Could you check a few things on this model? Use its own coordinates, in mm. A direction names the side the tool comes from. Give positions to 0.01 mm unless a question says otherwise; leave off trailing zeros. Loops run counter-clockwise (first coordinate to the right, second up) from the corner with the lowest first, then second, coordinate; pieces in that order, holes last. Notation, with made-up numbers: M -31,85 L 28,85 A34 ccw 28,118 Z; hole C -1,11 d6. An arc over 180 degrees is marked long. Write each question's results on one line, items separated by ' | '. Start each with the question number.
from build123d import *

# Parameters (mm, degrees)
SKETCH_1_W      = 23
SKETCH_1_H      = 20
SKETCH_1_H_2    = 12
SKETCH_1_R      = 1.5
SKETCH_1_W_2    = 19
SKETCH_1_R_2    = 1
EXTRUDE_1_DEPTH = 4
FILLET_1_R      = 3
CHAMFER_1_SIZE  = 15
FILLET_2_R      = 5


with BuildPart() as part:
    # 草图1 → 凸台-拉伸1 (new body)
    # profile 1 of 3: a face of its own
    with BuildSketch(Plane(origin=(0, 0, 0), x_dir=(1, 0, 0), z_dir=(0, 1, 0))):
        with Locations((51.5, 0)):
            Rectangle(SKETCH_1_W, SKETCH_1_H)
    # profile 2 of 3: a face of its own
    with BuildSketch(Plane(origin=(0, 0, 0), x_dir=(1, 0, 0), z_dir=(0, 1, 0))):
        with Locations((51.5, 16)):
            Rectangle(SKETCH_1_W, SKETCH_1_H_2)
        with Locations(Location((56, 18, 0), (0, 0, 270))):
            Circle(SKETCH_1_R, mode=Mode.SUBTRACT)
        with Locations(Location((48, 18, 0), (0, 0, 270))):
            Circle(SKETCH_1_R, mode=Mode.SUBTRACT)
    # profile 3 of 3: a face of its own
    with BuildSketch(Plane(origin=(0, 0, 0), x_dir=(1, 0, 0), z_dir=(0, 1, 0))):
        with Locations((30.5, 0)):
            Rectangle(SKETCH_1_W_2, SKETCH_1_H)
        with Locations(Location((24, -4, 0), (0, 0, 270))):
            Circle(SKETCH_1_R_2, mode=Mode.SUBTRACT)
        with Locations(Location((36, -4, 0), (0, 0, 270))):
            Circle(SKETCH_1_R_2, mode=Mode.SUBTRACT)
        with Locations(Location((24, 4, 0), (0, 0, 270))):
            Circle(SKETCH_1_R_2, mode=Mode.SUBTRACT)
        with Locations(Location((36, 4, 0), (0, 0, 270))):
            Circle(SKETCH_1_R_2, mode=Mode.SUBTRACT)
    extrude(amount=EXTRUDE_1_DEPTH)

    # 圆角1
    fillet_1_edges = [part.edges().sort_by_distance(p)[0] for p in [
        (21, 2, 10),
        (21, 2, -10),
        (40, 2, -10),
        (40, 2, -22),
        (63, 2, -22),
    ]]
    fillet(fillet_1_edges, radius=FILLET_1_R)

    # 倒角1
    chamfer_1_edges = [part.edges().sort_by_distance(p)[0] for p in [
        (63, 2, 10),
    ]]
    chamfer(chamfer_1_edges, length=CHAMFER_1_SIZE)

    # 圆角2
    fillet_2_edges = [part.edges().sort_by_distance(p)[0] for p in [
        (63, 2, -5),
        (48, 2, 10),
    ]]
    fillet(fillet_2_edges, radius=FILLET_2_R)


solid = part.part
1) If we section it at B-B on z = -18: Write out the boundary of the cut face in (x, y), plus the area to 3 significant figures.
2) Thinking about a two-plate mould opening in Z: for faces 3 (the face through (40, 2, -16)), 4 (the face through (37, 2, 4)), 5 (the face through (21.86, 2.03, 9.1)), 6 (the face through (46.536, 1.972, -18.325)), which applies, pulls with the +Z half, pulls with the -Z half, needs draft (parallel to the pull), parting line crosses it, or undercut?
3) If we section it at A-A on x = 56: Write out the boundary of the cut face in (y, z).
4) If we section it at D-D on y = 1.8: Write out the boundary of the cut face in (x, z).
5) Which directions (+Z, -Z, +X, -X, +Y, -Y) give clear straight access to the entire face, cutting with the end or side of a thin tool? Please do faces 1 (the face through (42, 0, -6)), 2 (the face through (30, 2, -10)).
6) Please list where these lines run through material, in increasing order: line 1 (X direction, y = 2.45, z = -18); line 2 (X direction, y = 1, z = -4); line 3 (X direction, y = 2.4, z = -14.5). Write a range as from..to.
7) I'm going to push a flat-ended pin straight in: P1, Ø3.5, axis at x = 56, z = -18, coming from the -Y side. Where does the tip first touch, or does it pass through?
8) If we section it at C-C on x = 36: Write out the boundary of the cut face in (y, z).
Calculated:
1) outline: M 40,0 L 46.5,0 L 46.5,4 L 40,4 Z; M 49.5,0 L 54.5,0 L 54.5,4 L 49.5,4 Z; M 57.5,0 L 63,0 L 63,4 L 57.5,4 Z | area: 68.0 mm2
2) face 3: needs draft | face 4: undercut | face 5: pulls with the +Z half | face 6: undercut
3) outline: M 0,-22 L 4,-22 L 4,-19.5 L 0,-19.5 Z; M 0,-16.5 L 4,-16.5 L 4,2 L 0,2 Z
4) outline: M 21,-7 A3 ccw 24,-10 L 37,-10 A3 cw 40,-13 L 40,-19 A3 ccw 43,-22 L 60,-22 A3 ccw 63,-19 L 63,-7.07 A5 ccw 61.54,-3.54 L 49.46,8.54 A5 ccw 45.93,10 L 24,10 A3 ccw 21,7 Z; hole C 24,-4 d2; hole C 24,4 d2; hole C 36,-4 d2; hole C 36,4 d2; hole C 48,-18 d3; hole C 56,-18 d3
5) face 1: +Z, -Z, +X, -X, -Y | face 2: -Z, -X, +Y, -Y
6) line 1: x = 40..46.5, 49.5..54.5, 57.5..63 | line 2: x = 21..23, 25..35, 37..61.95 | line 3: x = 40..63
7) P1: stops at y = 0
8) outline: M 0,-10 L 4,-10 L 4,-5 L 0,-5 Z; M 0,-3 L 4,-3 L 4,3 L 0,3 Z; M 0,5 L 4,5 L 4,10 L 0,10 Z
